Could you check a few things on this model? Use its own coordinates, in mm. Face numbers are marked on the shaded views. A direction names the side the tool comes from. Coordinates: 2 decimals unless noted, no trailing zeros. Loops run counter-clockwise (first coordinate to the right, second up) from the corner with the lowest first, then second, coordinate; pieces in that order, holes last.
1) Thinking about a two-plate mould opening in Y: for the marked faces 4, 5 and 6, which applies, released by +Y, released by -Y, zero draft, split by the parting line, or undercut?
2) Imagine slicing it at C-C on x = -39. Please give me the cut outline in (y, z).
3) Imagine slicing it at B-B on y = 174. Please give me the cut outline in (x, z), plus the area to 3 significant figures.
4) Will these pins go through, and if not, where does the flat tip stop? P1, Ø5.5, axis at y = 178.5, z = 126.5, coming from the +X side; P2, Ø1.5, axis at x = -68.5, z = 71, coming from the -Y side; P3, Ø6.5, axis at x = -162, y = 189.5, coming from the +Z side.
5) Imagine slicing it at D-D on z = 197.5. Please give me the cut outline in (x, y).
6) For the marked faces 1, 2 and 3, which set-ups out of +Z, -Z, +X, -X, +Y, -Y let a thin tool reach every point of the face, with its end or its side?
7) Imagine slicing it at A-A on z = 120. Please give me the cut outline in (x, y).
8) If I drill on line 1 along Y through (x, z) = (-71, 33.5); line 2 along Y through (x, z) = (-99, 56.5); line 3 along X through (y, z) = (288.5, 143), over which ranges is the centre line in solid material (lowest first)?
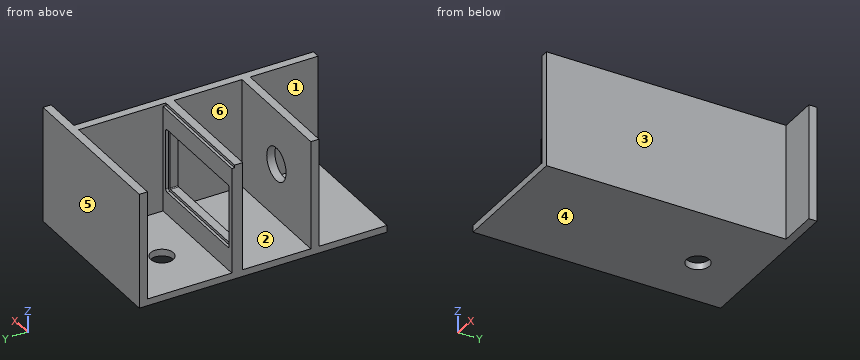
Autodesk Inventor part; units mm, degrees
ref_plane "YZ Plane" through (0, 0, 0) normal (1, 0, 0) x (0, 1, 0)
ref_plane "XZ Plane" through (0, 0, 0) normal (0, 1, 0) x (-1, 0, 0)
ref_plane "XY Plane" through (0, 0, 0) normal (0, 0, 1) x (1, 0, 0)
sketch "Skizze1" plane through (0, 0, 0) normal (1, 0, 0) x (0, 1, 0)
  line L0 (0, 0) -> (18, 0)
  line L1 (18, 0) -> (18, 240)
  line L2 (18, 240) -> (0, 240)
  line L3 (0, 240) -> (0, 0)
  line L4 (378, 0) -> (-150, 0)
  line L5 (-150, -15) -> (378, -15)
  line L6 (378, -15) -> (378, 0)
  line L7 (378, -15) -> (378, 240)
  line L8 (378, 240) -> (396, 240)
  line L9 (396, 240) -> (396, -15)
  line L10 (396, -15) -> (378, -15)
  line L11 (-150, 0) -> (-150, -15)
  line L12 (186, 0) -> (168, 0)
  line L13 (168, 0) -> (168, 240)
  line L14 (168, 240) -> (186, 240)
  line L15 (186, 240) -> (186, 0)
  dimension "d0" = 18
  dimension "d1" = 15
  dimension "d2" = 18
  dimension "d5" = 255
  dimension "d6" = 360
  dimension "d23" = 150
  dimension "d49" = 18
  dimension "d50" = 150
  dimension "d51" = 192
  dimension "d52" = 255
extrude "Extrusion1" add sketch "Skizze1" against normal blind 260
extrude "Extrusion7" add sketch "Skizze1" along normal blind 104 contours L6 L7 L8 L9 L10
sketch "Skizze2" plane through (0, 0, 0) normal (0, -1, 0) x (1, 0, 0)
  line L0 (0, 0) -> (-260, 0)
  line L1 (0, 240) -> (-260, 240)
  circle A0 centre (-130, 120) radius 36.5
  line L2 (-130, 240) -> (-130, 0) construction
  point P0 (240, 0)
  dimension "d9" = 73
extrude "Extrusion2" cut sketch "Skizze2" against normal up to surface (18 mm away)
sketch "Skizze4" plane through (0, 18, 0) normal (0, 0, 1) x (1, 0, 0)
  circle A0 centre (-140.0937, 257.9889) radius 25
  ellipse E0 centre (-140.0937, 257.9889) end of major axis (-140.0937, 283.4889) minor radius 25.5
  dimension "d16" = 50
extrude "Extrusion4" cut sketch "Skizze4" against normal up to surface (15 mm away) contours A0
sketch "Skizze6" plane through (0, 0, 0) normal (1, 0, 0) x (0, 0, -1)
  line L0 (15, -150) -> (15, 378)
  line L1 (-240, 378) -> (15, 378)
  line L2 (15, 378) -> (15, -150)
  line L3 (15, -150) -> (-240, -150)
  line L4 (-240, -150) -> (-240, 378)
  line L5 (15, 396) -> (15, 378)
  line L6 (15, 378) -> (15, -150)
  line L7 (15, -150) -> (0, -150)
  line L8 (0, 0) -> (-240, 0)
  line L9 (-240, 0) -> (-240, 18)
  line L10 (-240, 18) -> (0, 18)
  line L11 (0, 186) -> (0, 378)
  line L12 (0, 378) -> (-240, 378)
  line L13 (-240, 378) -> (-240, 396)
  line L14 (-240, 396) -> (15, 396)
  line L15 (15, 378) -> (0, 378)
  line L16 (-240, 168) -> (-240, 186)
  line L17 (-240, 186) -> (0, 186)
  line L18 (0, 18) -> (0, 168)
  line L19 (0, 168) -> (-240, 168)
  line L20 (0, -150) -> (0, 0)
extrude "Extrusion8" add sketch "Skizze6" along normal blind 18
sketch "Skizze9" plane through (-260, 186, 240) normal (0, 1, 0) x (1, 0, 0)
  line L0 (260, 240) -> (0, 240)
  line L1 (260, 0) -> (0, 0)
  line L2 (250, 185) -> (250, 55)
  line L3 (245, 50) -> (15, 50)
  line L4 (10, 55) -> (10, 185)
  line L5 (15, 190) -> (245, 190)
  line L6 (250, 190) -> (10, 50) construction
  line L7 (250, 50) -> (10, 190) construction
  arc A0 (250, 185) -> (245, 190) centre (245, 185) ccw
  arc A1 (15, 190) -> (10, 185) centre (15, 185) ccw
  arc A2 (10, 55) -> (15, 50) centre (15, 55) ccw
  arc A3 (245, 50) -> (250, 55) centre (245, 55) ccw
  line L8 (14, 184) -> (14, 56)
  line L9 (16, 54) -> (244, 54)
  line L10 (246, 56) -> (246, 184)
  line L11 (244, 186) -> (16, 186)
  line L12 (14, 186) -> (246, 54) construction
  line L13 (14, 54) -> (246, 186) construction
  arc A4 (244, 54) -> (246, 56) centre (244, 56) ccw
  arc A5 (14, 56) -> (16, 54) centre (16, 56) ccw
  arc A6 (16, 186) -> (14, 184) centre (16, 184) ccw
  arc A7 (246, 184) -> (244, 186) centre (244, 184) ccw
  line L14 (244, 182) -> (244, 58)
  line L15 (242, 56) -> (18, 56)
  line L16 (16, 58) -> (16, 182)
  line L17 (18, 184) -> (242, 184)
  line L18 (244, 184) -> (16, 56) construction
  line L19 (244, 56) -> (16, 184) construction
  arc A8 (242, 56) -> (244, 58) centre (242, 58) ccw
  arc A9 (16, 58) -> (18, 56) centre (18, 58) ccw
  arc A10 (18, 184) -> (16, 182) centre (18, 182) ccw
  arc A11 (244, 182) -> (242, 184) centre (242, 182) ccw
  line L20 (130, 0) -> (130, 240) construction
  line L21 (0, 240) -> (260, 240)
  line L22 (260, 240) -> (260, 0)
  line L23 (260, 0) -> (0, 0)
  line L24 (0, 0) -> (0, 240)
  line L25 (260, 240) -> (260, 0)
  line L26 (0, 0) -> (260, 0)
  line L27 (260, 0) -> (260, 6)
  line L28 (260, 6) -> (0, 6)
  line L29 (0, 6) -> (0, 0)
  point P0 (130, 120)
  dimension "d53" = 140
  dimension "d54" = 240
  dimension "d55" = 5
  dimension "d56" = 232
  dimension "d57" = 132
  dimension "d58" = 2
  dimension "d59" = 128
  dimension "d60" = 228
  dimension "d61" = 2
  dimension "d67" = 6
extrude "Extrusion11" cut sketch "Skizze9" against normal up to surface (18 mm away) contours L14 A8 L15 A9 L16 A10 L17 A11
extrude "Extrusion12" add sketch "Skizze9" along normal blind 6 contours L22 L28 L24 L0
equation "\"d0\" = case_thickness"
equation "\"d1\" = inner_thickness"
equation "\"d2\" = case_thickness"
equation "\"d5\" = inner_depth"
equation "\"d49\" = case_thickness"
equation "\"d52\" = inner_depth"
equation "\"d7\" = inner_width"
equation "\"d26\" = -2 * case_thickness + case_width - inner_width"
equation "\"d10\" = case_width - 2 * case_thickness"
equation "\"d16\" = ht_diameter"
equation "\"d17\" = case_width - 2 * case_thickness"
equation "\"d28\" = case_thickness"
equation "\"d67\" = mdf_thickness"
equation "\"d65\" = mdf_thickness"
equation "\"kg_thickness\" = 4.9"
equation "\"ht_diameter\" = 50"
equation "\"ht_thickness\" = 1.9"
equation "\"case_thickness\" = 18"
equation "\"inner_thickness\" = 15"
equation "\"gap_fit\" = 0.1"
equation "\"gap_slide\" = 0.2"
equation "\"gap_air\" = 1"
equation "\"bore_diameter\" = 73"
equation "\"mdf_thickness\" = 6"
equation "\"tape_width\" = 15"
equation "\"tape_thickness\" = 3"
equation "\"inner_depth\" = 255"
equation "\"inner_width\" = 260"
properties part number "Korpus_Einbau"
Filled in:
1. face 4: zero draft
1. face 5: released by +Y
1. face 6: undercut
2. outline: (-150, -15) - (396, -15) - (396, 240) - (378, 240) - (378, 0) - (192, 0) - (192, 50) - (186, 50) - (186, 56) - (168, 56) - (168, 0) - (18, 0) - (18, 240) - (0, 240) - (0, 0) - (-150, 0) - close; (168, 184) - (186, 184) - (186, 190) - (192, 190) - (192, 234) - (186, 234) - (186, 240) - (168, 240) - close
3. outline: (-260, -15) - (18, -15) - (18, 240) - (-260, 240) - close; hole (-244, 58) arc R2 ccw to (-242, 56) - (-18, 56) arc R2 ccw to (-16, 58) - (-16, 182) arc R2 ccw to (-18, 184) - (-242, 184) arc R2 ccw to (-244, 182) - close
3. area: 41,700 mm2
4. P1: stops at x = 18
4. P2: stops at y = 0
4. P3: stops at z = 234
5. outline: (-260, 0) - (0, 0) - (0, -150) - (18, -150) - (18, 378) - (104, 378) - (104, 396) - (-260, 396) - (-260, 378) - (0, 378) - (0, 192) - (-260, 192) - (-260, 168) - (0, 168) - (0, 18) - (-260, 18) - close
6. face 1: +Z, -X, -Y
6. face 2: +Z, -X
6. face 3: +Z, -Z, +X, -Y
7. outline: (-260, 0) - (-166.5, 0) - (-166.5, 18) - (-260, 18) - close; (-260, 168) - (-244, 168) - (-244, 186) - (-250, 186) - (-250, 192) - (-260, 192) - close; (-260, 378) - (0, 378) - (0, 192) - (-10, 192) - (-10, 186) - (-16, 186) - (-16, 168) - (0, 168) - (0, 18) - (-93.5, 18) - (-93.5, 0) - (0, 0) - (0, -150) - (18, -150) - (18, 378) - (104, 378) - (104, 396) - (-260, 396) - close
8. line 1: y = 0 to 18, 168 to 192, 378 to 396
8. line 2: y = 0 to 18, 378 to 396
8. line 3: x = 0 to 18
